The model under review builds one solid part; all positions refer to its coordinate system, in mm. A direction names the side the tool comes from. Give positions to 0.01 mm unless a question says otherwise; leave off trailing zeros. Order: outer loops, then holes, each group sorted by start corner. A loop starts at its lowest first (then second) coordinate and runs counter-clockwise, first axis right, second up.
Autodesk Inventor part; units mm, degrees
ref_plane "YZ Plane" through (0, 0, 0) normal (1, 0, 0) x (0, 1, 0)
ref_plane "XZ Plane" through (0, 0, 0) normal (0, 1, 0) x (-1, 0, 0)
ref_plane "XY Plane" through (0, 0, 0) normal (0, 0, 1) x (1, 0, 0)
sketch "Sketch1" plane through (0, 0, 0) normal (0, 0, 1) x (1, 0, 0)
  line L0 (48, -32) -> (-48, -32)
  line L1 (-48, -32) -> (-48, 32)
  line L2 (-48, 32) -> (48, 32)
  line L3 (48, 32) -> (48, -32)
  line L4 (48, -32) -> (-48, 32) construction
  line L5 (-48, -32) -> (48, 32) construction
  point P0 (0, 0)
  dimension "d0" = 96
  dimension "d1" = 64
extrude "Extrusion1" add sketch "Sketch1" along normal blind 16
sketch "Sketch2" plane through (0, 0, 16) normal (0, 0, 1) x (1, 0, 0)
  point P0 (0, 0)
sketch "Sketch3" plane through (0, 0, 16) normal (0, 0, 1) x (1, 0, 0)
  line L0 (48, 32) -> (-48, 32)
  line L1 (-48, 32) -> (-32, 32)
  line L2 (-32, 32) -> (-32, -32)
  line L3 (-32, -32) -> (-48, -32)
  line L4 (-48, -32) -> (-48, 32)
  line L5 (-48, -32) -> (48, -32)
  point P0 (0, 0)
  dimension "d4" = 16
extrude "Extrusion2" add sketch "Sketch3" along normal blind 48
fillet "Fillet1" radius 32 1 edges at (-40, -32, 64)
sketch "Sketch4" plane through (-48, 32, 0) normal (0, 1, 0) x (1, 0, 0)
  line L0 (16, -16) -> (96, -16)
  line L1 (16, -16) -> (56, -16)
  line L2 (56, -16) -> (56, -44)
  line L3 (16, -44) -> (16, -16)
  arc A0 (48, -44) -> (24, -44) centre (36, -44) ccw
  line L4 (56, -44) -> (48, -44)
  line L5 (24, -44) -> (16, -44)
  point P0 (48, 0)
  dimension "d8" = 40
  dimension "d9" = 28
  dimension "d10" = 24
extrude "Extrusion3" add sketch "Sketch4" against normal blind 42
sketch "Sketch5" plane through (-48, 32, 0) normal (0, 1, 0) x (1, 0, 0)
  line L0 (56, -16) -> (56, -44)
  line L1 (56, -44) -> (56, -16)
  line L2 (96, -16) -> (56, -16)
  line L3 (56, -16) -> (96, -16)
  line L4 (96, -16) -> (56, -44)
  point P0 (48, 0)
extrude "Extrusion4" add sketch "Sketch5" against normal blind 12
sketch "Sketch6" plane through (0, 0, 16) normal (0, 0, 1) x (1, 0, 0)
  line L0 (48, -32) -> (48, 20)
  line L1 (48, -16) -> (28, -16)
  arc A0 (28, 0) -> (28, -16) centre (28, -8) ccw
  line L2 (28, 0) -> (48, 0)
  line L3 (-32, -32) -> (48, -32)
  point P0 (0, 0)
  dimension "d15" = 20
  dimension "d16" = 16
  dimension "d17" = 16
extrude "Extrusion5" cut sketch "Sketch6" against normal blind 16
properties part number "Practical 1"
1. Draft analysis for pull direction X (two halves, no side actions). For faces 5 (the flat face through (48, 16, 8)), 6 (the cylindrical face through (-12, 11, 32)), 7 (the flat face through (1, -32, 9)), state which applies: pulls with the +X half, pulls with the -X half, needs draft (parallel to the pull), parting line crosses it, or undercut.
2. Take a section at B-B (y = 17). Write out the cut boundary in (x, z).
3. Take a section at D-D (y = -5.5). Write out the cut boundary in (x, z).
4. For faces 1 (the flat face through (38, 0, 8)), 2 (the flat face through (-40, 16, 64)), 3 (the flat face through (8, 5, 30)), 4 (the flat face through (-28, 11, 44)), list the 3-axis set-ups (+Z, -Z, +X, -X, +Y, -Y) from which the entire face can be reached by the end or side of a thin tool; tool diameter is ignored.
5. To check wall thickness, follow line 1 (Z direction, x = -31, y = 5); line 2 (X direction, y = -8, z = 55); line 3 (Y direction, x = 24, z = 26). State the ranges of each line that lie inside material, in increasing order.
6. Take a section at A-A (z = 37). Write out the cut boundary in (x, y), and give its area (3 significant figures).
7. Take a section at C-C (x = 4). Write out the cut boundary in (y, z), and give its area (3 significant figures).
8. Insertion check: pin 1 (22.5 mm diameter, centred on x = 32, z = 29.5, fed in from -Y); pin 2 (4 mm diameter, centred on x = 5, y = 8.5, fed in from +Z); pin 3 (14 mm diameter, centred on x = -17, z = 26.5, fed in from -Y). Each pin has a flat end and moves straight along its axis. Give the tip position at first contact, or say it passes through.
Answer:
1. face 5: pulls with the +X half
1. face 6: undercut
1. face 7: needs draft
2. outline: (-48, 0) - (48, 0) - (48, 16) - (8, 16) - (8, 44) - (0, 44) arc R12 cw to (-24, 44) - (-32, 44) - (-32, 64) - (-48, 64) - close
3. outline: (-48, 0) - (20.4, 0) - (20.4, 16) - (8, 16) - (8, 44) - (0, 44) arc R12 cw to (-24, 44) - (-32, 44) - (-32, 63.52) - (-48, 63.52) - close
4. face 1: +Z, -Z, +X
4. face 2: +Z, +X, -X, +Y, -Y
4. face 3: +Z, +X, -Y
4. face 4: +Z, +X, +Y, -Y
5. line 1: z = 0 to 44
5. line 2: x = -48 to -32
5. line 3: y = 20 to 32
6. outline: (-48, -31.61) - (-32, -31.61) - (-32, -10) - (-21.75, -10) - (-21.75, 32) - (-48, 32) - close; (-2.25, -10) - (8, -10) - (8, 20) - (18, 20) - (18, 32) - (-2.25, 32) - close
6. area: 2,000 mm2
7. outline: (-32, 0) - (32, 0) - (32, 44) - (-10, 44) - (-10, 16) - (-32, 16) - close
7. area: 2,200 mm2
8. pin 1: stops at y = 20
8. pin 2: stops at z = 44
8. pin 3: stops at y = -10
